from build123d import *

# Parameters (mm, degrees)
F0_R     = 4
F1_DEPTH = 6.25
F0_R_2   = 9.7
F2_DEPTH = 1.75
F3_SIZE  = 0.75
F4_R     = 0.5


with BuildPart() as f1:
    # F0 (on Front) → F1 (new body)
    with BuildSketch(Plane.XZ):
        Circle(F0_R)
    extrude(amount=F1_DEPTH)

    # F0 (on Front) → F2 (join)
    with BuildSketch(Plane.XZ):
        Circle(F0_R_2)
        Circle(F0_R, mode=Mode.SUBTRACT)
    extrude(amount=F2_DEPTH)

    # F3
    f3_edges = [f1.edges().sort_by_distance(p)[0] for p in [
        (-9.7, -1.75, 0),
    ]]
    chamfer(f3_edges, length=F3_SIZE)

    # F4
    f4_edges = [f1.edges().sort_by_distance(p)[0] for p in [
        (-9.7, 0, 0),
    ]]
    fillet(f4_edges, radius=F4_R)


solid = f1.part
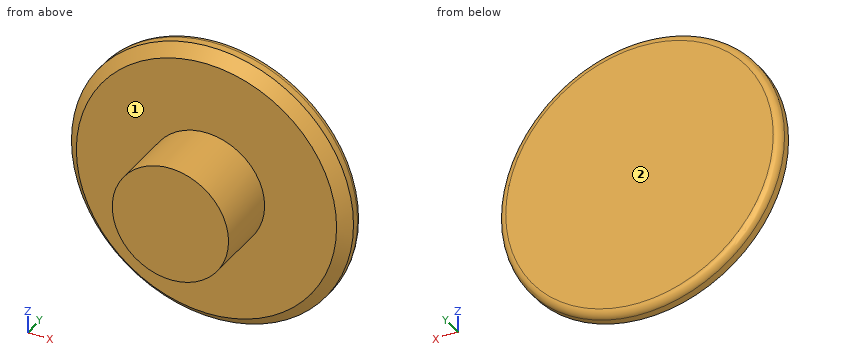
Source: CAD feature listing. Evaluate the final solid. Frame: model axes, mm. Face numbers are marked on the shaded views. A direction names the side the tool comes from. Round coordinates to 2 decimals unless told otherwise and drop trailing zeros. Loops run counter-clockwise (first coordinate to the right, second up) from the corner with the lowest first, then second, coordinate; pieces in that order, holes last.
Q1. Section A-A, the plane x = 0. Return loops of the section in (y, z).
Q2. Access query for the marked faces 1 and 2. Directions: +Z, -Z, +X, -X, +Y, -Y. A direction counts if a zero-diameter tool reaches every point of the face in a straight line with its end or side. Return the directions, or none.
Q3. First-contact query: P1, Ø3, axis at x = 3, z = -7, coming from the -Y side; P2, Ø6, axis at x = 6, z = -2, coming from the -Y side; P3, Ø2, axis at y = -2, z = -7, coming from the +X side. Flat tips, straight axial feed; report the tip coordinate or a pass-through.
Q4. Section C-C, the plane y = -4. Return loops of the section in (x, z).
Q5. Ray query, line 1 (Y direction, x = -6, z = -3.5); line 2 (X direction, y = -4.5, z = 1.75); line 3 (X direction, y = -3.5, z = 3). Return the intervals inside material, ascending.
Q6. Section B-B, the plane z = 0. Return loops of the section in (x, y).
Solutions:
1. outline: (-6.25, -4) - (-1.75, -4) - (-1.75, -8.95) - (-1, -9.7) - (-0.5, -9.7) arc R0.5 ccw to (0, -9.2) - (0, 9.2) arc R0.5 ccw to (-0.5, 9.7) - (-1, 9.7) - (-1.75, 8.95) - (-1.75, 4) - (-6.25, 4) - close
2. face 1: -Y
2. face 2: +Z, -Z, +X, -X, +Y
3. P1: stops at y = -1.75
3. P2: stops at y = -6.25
3. P3: stops at x = 7.02
4. outline: circle Ø8 at (0, 0)
5. line 1: y = -1.75 to 0
5. line 2: x = -3.6 to 3.6
5. line 3: x = -2.65 to 2.65
6. outline: (-9.7, -1) - (-8.95, -1.75) - (-4, -1.75) - (-4, -6.25) - (4, -6.25) - (4, -1.75) - (8.95, -1.75) - (9.7, -1) - (9.7, -0.5) arc R0.5 ccw to (9.2, 0) - (-9.2, 0) arc R0.5 ccw to (-9.7, -0.5) - close
